Print and shaded views of the part. All mm, measured from the part's lowest x, y and z. A direction names the side the tool comes from. Round coordinates to 2 decimals unless told otherwise and drop trailing zeros. Loops run counter-clockwise (first coordinate to the right, second up) from the corner with the lowest first, then second, coordinate; pieces in that order, holes last. Notation, with made-up numbers: (-20, 8.25) - (16, 8.25) arc R18 cw to (16, 38.25) - close; hole circle Ø3 at (-32, 44.25). An arc over 180 degrees is marked (long way). Answer as a JSON object with one key per item and string values.
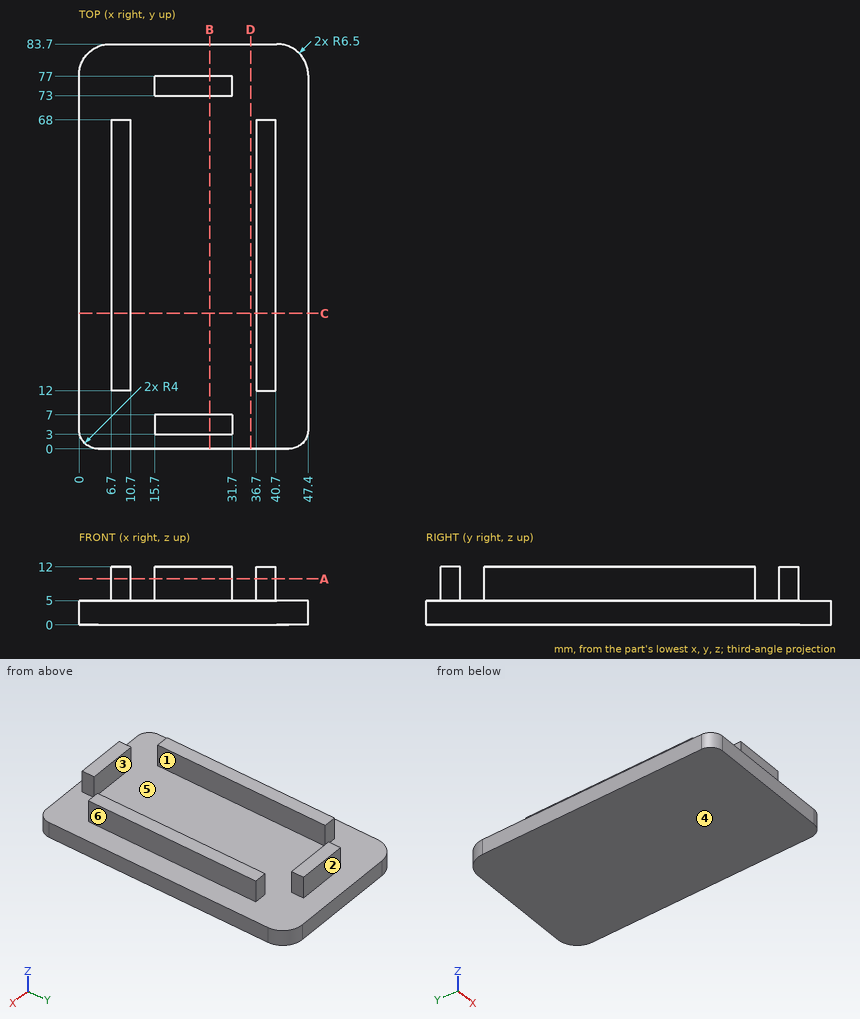
1) Drop flat-ended pins along their axis: P1, Ø5.5, axis at y = 32, z = 9, coming from the -X side; P2, Ø2, axis at y = 4.5, z = 8, coming from the +X side; P3, Ø3, axis at x = 38.5, z = 8, coming from the +Y side; P4, Ø8, axis at x = 26.5, y = 10, coming from the -Z side. Give the stop position or say it passes through.
Values follow:
{"P1": "x = 6.7", "P2": "x = 31.7", "P3": "y = 68", "P4": "z = 0"}
2) Slice it at A-A on z = 9.5. List the corners of the cut face in (x, y), then the cut area to 3 significant figures.
Values follow:
{"outline": "(6.7, 12) - (10.7, 12) - (10.7, 68) - (6.7, 68) - close; (15.7, 3) - (31.7, 3) - (31.7, 7) - (15.7, 7) - close; (15.7, 73) - (31.7, 73) - (31.7, 77) - (15.7, 77) - close; (36.7, 12) - (40.7, 12) - (40.7, 68) - (36.7, 68) - close", "area": "576 mm²"}
3) Slice it at D-D on x = 35.5. List the corners of the cut face in (y, z), then the cut area to 4 significant figures.
Values follow:
{"outline": "(0, 0) - (83.7, 0) - (83.7, 5) - (0, 5) - close", "area": "418.5 mm²"}
4) Slice it at B-B on x = 27. List the corners of the cut face in (y, z).
Values follow:
{"outline": "(0, 0) - (83.7, 0) - (83.7, 5) - (77, 5) - (77, 12) - (73, 12) - (73, 5) - (7, 5) - (7, 12) - (3, 12) - (3, 5) - (0, 5) - close"}
5) Tool access for the marked faces 1, 2 and 3: list every direction of +Z, -Z, +X, -X, +Y, -Y with a clear straight run to the whole face (end or side of a thin tool).
Values follow:
{"face 1": "+Z, +Y, -Y", "face 2": "+Z, +X, -X, +Y", "face 3": "+Z, +X, -X"}
6) Probe probe 1 along X at (y, z) = (16.5, 9.5); probe 2 along Y at (x, z) = (23, 11.75); probe 3 along Z at (x, y) = (17, 31.5). List the from-to ranges inside material, lowest first.
Values follow:
{"probe 1": "6.7 to 10.7, 36.7 to 40.7", "probe 2": "3 to 7, 73 to 77", "probe 3": "0 to 5"}
7) Slice it at C-C on y = 28. List the corners of the cut face in (x, z), then the cut area to 3 significant figures.
Values follow:
{"outline": "(0, 0) - (47.4, 0) - (47.4, 5) - (40.7, 5) - (40.7, 12) - (36.7, 12) - (36.7, 5) - (10.7, 5) - (10.7, 12) - (6.7, 12) - (6.7, 5) - (0, 5) - close", "area": "293 mm²"}
8) Two-plate mould, pull along X, no slides. Class the marked faces 4, 5 and 6: pulls with the +X half, pulls with the -X half, needs draft (parallel to the pull), parting line crosses it, or undercut.
Values follow:
{"face 4": "needs draft", "face 5": "undercut", "face 6": "pulls with the +X half"}
